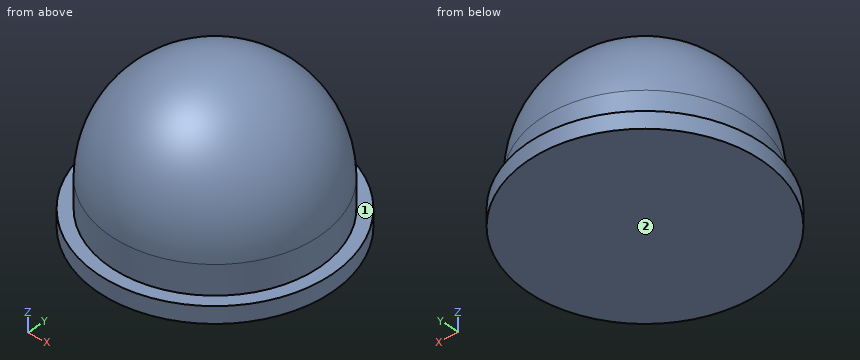
from build123d import *

# Parameters (mm, degrees)
SKETCH1_R           = 12.5
BOSS_EXTRUDE1_DEPTH = 16
FILLET1_R           = 12.5
SKETCH2_R           = 14
BOSS_EXTRUDE2_DEPTH = 2


with BuildPart() as part:
    # Sketch1 → Boss-Extrude1 (new body)
    with BuildSketch(Plane.XY):
        Circle(SKETCH1_R)
    extrude(amount=BOSS_EXTRUDE1_DEPTH)

    # Fillet1
    fillet1_edges = [part.edges().sort_by_distance(p)[0] for p in [
        (-12.5, 0, 16),
    ]]
    fillet(fillet1_edges, radius=FILLET1_R)

    # Sketch2 → Boss-Extrude2 (add)
    with BuildSketch(Plane(origin=(0, 0, 0), x_dir=(-1, 0, 0), z_dir=(0, 0, -1))):
        Circle(SKETCH2_R)
    extrude(amount=BOSS_EXTRUDE2_DEPTH)


solid = part.part
Part model, mm, in its own coordinate system. Face numbers are marked on the shaded views. A direction names the side the tool comes from. Round coordinates to 2 decimals unless told otherwise and drop trailing zeros. Order: outer loops, then holes, each group sorted by start corner. A loop starts at its lowest first (then second) coordinate and runs counter-clockwise, first axis right, second up. Notation, with made-up numbers: (39.5, -35) -> (65.5, -35) arc R22 ccw to (65.5, -20) -> close; hole circle Ø7 at (26, 59.25). An arc over 180 degrees is marked (long way). Put each result on its own line as item: value.
Q1. Tool access for the marked faces 1 and 2: list every direction of +Z, -Z, +X, -X, +Y, -Y with a clear straight run to the whole face (end or side of a thin tool).
From the geometry:
face 1: +Z
face 2: -Z, +X, -X, +Y, -Y
Q2. Pin check, flat tips, straight feed: pin 1 Ø8 at (x, z) = (10.5, 4.5) entering from +Y; pin 2 Ø3 at (y, z) = (3.5, 0.5) entering from +X; pin 3 Ø10 at (y, z) = (-8, 14) entering from +X. Stop position of each tip, or through.
From the geometry:
pin 1: stops at y = 10.65
pin 2: stops at x = 13.84
pin 3: stops at x = 9.43
Q3. Band-saw the part on D-D (z = 13.5). Give the cut face in (x, y), and give its area (3 significant figures).
From the geometry:
outline: circle Ø15 at (0, 0)
area: 177 mm2
Q4. Wall check: line 1 (Z direction, x = -5.75, y = -11.5); line 2 (X direction, y = -6.25, z = 1.5); line 3 (Y direction, x = -8.5, z = 11). Give the ranges that are in metal, low to high. Write a range as [from, to].
From the geometry:
line 1: z = [-2, 0]
line 2: x = [-10.83, 10.83]
line 3: y = [-5.27, 5.27]
Q5. Band-saw the part on A-A (y = 0). Give the cut face in (x, z).
From the geometry:
outline: (-14, -2) -> (14, -2) -> (14, 0) -> (12.5, 0) -> (12.5, 3.5) arc R12.5 ccw to (-12.5, 3.5) -> (-12.5, 0) -> (-14, 0) -> close
Q6. Band-saw the part on C-C (z = 2). Give the cut face in (x, y).
From the geometry:
outline: circle Ø25 at (0, 0)
